Check sheet for the modelled part. Datum: model origin and axes. Units: mm. A direction names the side the tool comes from. Coordinates: 2 decimals unless noted, no trailing zeros. Write each loop counter-clockwise with the first axis right and the second up, starting at its lowest first coordinate (ties: lowest second). Pieces come first, ordered by that corner, then holes. Notation, with made-up numbers: (85.25, 11.25) -> (132.25, 11.25) arc R22 cw to (132.25, 21.25) -> close; hole circle Ø5 at (-19.75, 76.5). An arc over 180 degrees is marked (long way). Put each result on its own line as item: value.
```python
from build123d import *

# Parameters (mm, degrees)
SKETCH1_W           = 3
SKETCH1_H           = 20
BOSS_EXTRUDE1_DEPTH = 10
SKETCH2_W           = 17
SKETCH2_H           = 17
BOSS_EXTRUDE2_DEPTH = 20
SKETCH3_R           = 4.25
CUT_EXTRUDE1_DEPTH  = 30.021543722
FILLET1_R           = 2


with BuildPart() as part:
    # Sketch1 → Boss-Extrude1 (new, symmetric)
    with BuildSketch(Plane(origin=(0, 0, 0), x_dir=(0, 0, -1), z_dir=(1, 0, 0))):
        with Locations((-1.5, 0)):
            Rectangle(SKETCH1_W, SKETCH1_H)
    extrude(amount=BOSS_EXTRUDE1_DEPTH, both=True)

    # Sketch2 → Boss-Extrude2 (add)
    with BuildSketch(Plane(origin=(0, 0, 0), x_dir=(-1, 0, 0), z_dir=(0, 0, -1))):
        Rectangle(SKETCH2_W, SKETCH2_H)
    extrude(amount=BOSS_EXTRUDE2_DEPTH)

    # Sketch3 → Cut-Extrude1 (cut, through all)
    with BuildSketch(Plane(origin=(8.5, 0, 0), x_dir=(0, 0, -1), z_dir=(1, 0, 0))):
        with Locations((10.5, 0)):
            Circle(SKETCH3_R)
    extrude(amount=-CUT_EXTRUDE1_DEPTH, mode=Mode.SUBTRACT)

    # Fillet1
    fillet1_edges = [part.edges().sort_by_distance(p)[0] for p in [
        (-10, 0, 3),
        (0, -10, 3),
        (0, 10, 3),
        (10, 0, 3),
    ]]
    fillet(fillet1_edges, radius=FILLET1_R)


solid = part.part
```
Q1. Mould release check, pull along Z, two halves, no side actions. Record for faces 1 (the flat face through (0, 0, 3)), 2 (the cylindrical face through (0.119, 3.584, -12.785)), 3 (the flat face through (-8.5, 0, -5)): released by +Z, released by -Z, zero draft, split by the parting line, or undercut.
Recorded:
face 1: released by +Z
face 2: undercut
face 3: zero draft
Q2. Cross-section at C-C (x = 5.25). Record the cut outline in (y, z), plus the area to 3 significant figures.
Recorded:
outline: (-10, 0) -> (-8.5, 0) -> (-8.5, -20) -> (8.5, -20) -> (8.5, 0) -> (10, 0) -> (10, 1) arc R2 ccw to (8, 3) -> (-8, 3) arc R2 ccw to (-10, 1) -> close; hole circle Ø8.5 at (0, -10.5)
area: 342 mm2
Q3. Depth check by flat-ended pin: P1, Ø4, axis at x = -6.5, z = -8, coming from the -Y side; P2, Ø1, axis at y = -1, z = -4, coming from the +X side. Enter the tip coordinate at first touch or a pass-through.
Recorded:
P1: stops at y = -8.5
P2: stops at x = 8.5
Q4. Cross-section at D-D (y = -7). Record the cut outline in (x, z).
Recorded:
outline: (-10, 0) -> (-8.5, 0) -> (-8.5, -20) -> (8.5, -20) -> (8.5, 0) -> (10, 0) -> (10, 1) arc R2 ccw to (8, 3) -> (-8, 3) arc R2 ccw to (-10, 1) -> close
Q5. Cross-section at B-B (z = -10.5). Record the cut outline in (x, y).
Recorded:
outline: (-8.5, -8.5) -> (8.5, -8.5) -> (8.5, -4.25) -> (-8.5, -4.25) -> close; (-8.5, 4.25) -> (8.5, 4.25) -> (8.5, 8.5) -> (-8.5, 8.5) -> close
Q6. Tool access check on faces 4 (the flat face through (0, -8.5, -10)), 5 (the flat face through (8.5, 0, -5)), 6 (the cylindrical face through (0.14, -9.4, 2.43)), 7 (the flat face through (0, 8.5, -10)). Record the directions out of +Z, -Z, +X, -X, +Y, -Y that give a thin tool (end or side, any length) a straight path to the whole face; none if there is none.
Recorded:
face 4: -Z, +X, -X, -Y
face 5: -Z, +X, +Y, -Y
face 6: +Z, +X, -X, -Y
face 7: -Z, +X, -X, +Y
Q7. Cross-section at A-A (y = 0). Record the cut outline in (x, z), plus the area to 3 significant figures.
Recorded:
outline: (-10, 0) -> (-8.5, 0) -> (-8.5, -6.25) -> (8.5, -6.25) -> (8.5, 0) -> (10, 0) -> (10, 1) arc R2 ccw to (8, 3) -> (-8, 3) arc R2 ccw to (-10, 1) -> close; (-8.5, -20) -> (8.5, -20) -> (8.5, -14.75) -> (-8.5, -14.75) -> close
area: 254 mm2
Q8. Material ranges on line 1 along Y through (x, z) = (5, -10.5); line 2 along X through (y, z) = (4, -14); line 3 along Y through (x, z) = (-5, -13.75), recorded low to high.
Recorded:
line 1: y = -8.5 to -4.25, 4.25 to 8.5
line 2: x = -8.5 to 8.5
line 3: y = -8.5 to -2.74, 2.74 to 8.5
